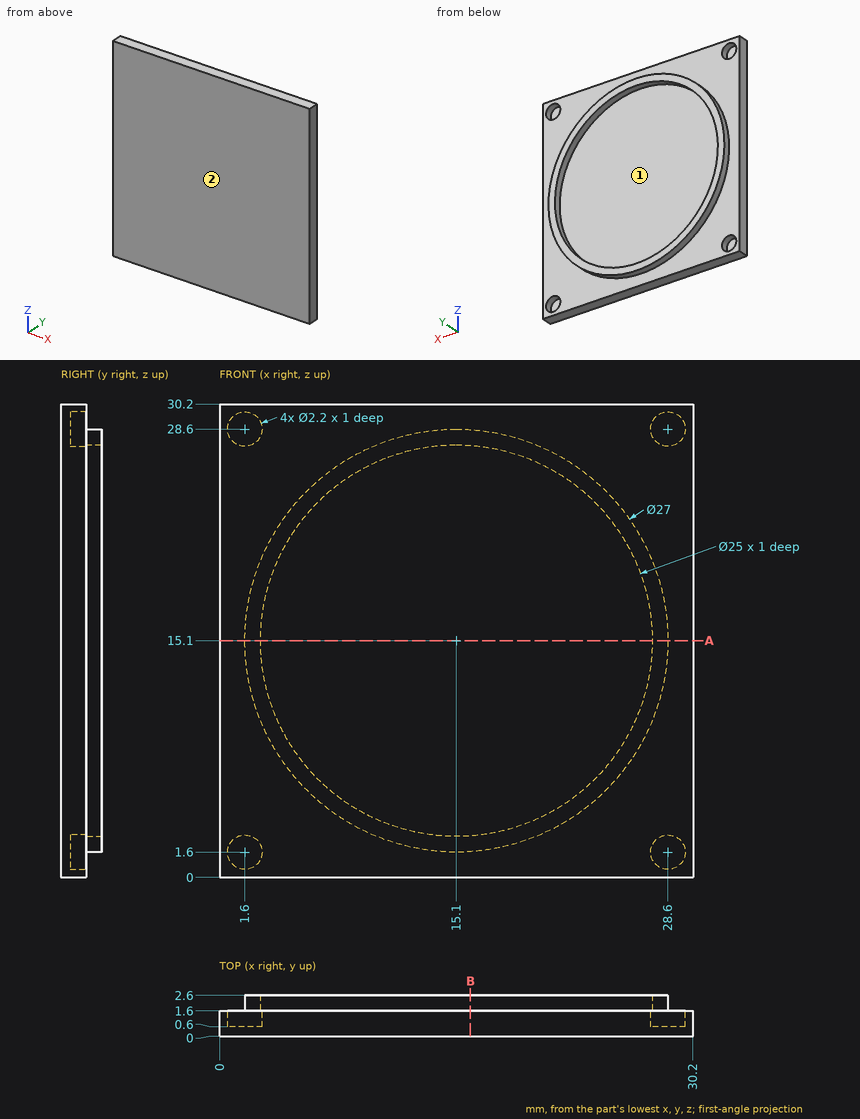
Geometry: see drawing. Coordinates: mm, zero at the bounding-box minimum. Coordinates: 2 decimals unless noted, no trailing zeros. Order: outer loops, then holes, each group sorted by start corner. A loop starts at its lowest first (then second) coordinate and runs counter-clockwise, first axis right, second up. Notation, with made-up numbers: (-16, 32) -> (7, 32) arc R14 ccw to (7, 37) -> close; hole circle Ø3 at (58, 33). An arc over 180 degrees is marked (long way). Write each question's results on one line, items separated by ' | '. Start each with the question number.
1) Cut plane B-B, the plane x = 16. Output: boundary loops of the cut face in (y, z), and give its area (3 significant figures).
2) Mould query, pull axis X, two halves, no side actions, for the marked faces 1 and 2. Classes: released by +X, released by -X, zero draft, split by the parting line, or undercut.
3) Cut plane A-A, the plane z = 15.1. Output: boundary loops of the cut face in (x, y).
4) Material intervals for line 1 along X through (y, z) = (1.1, 1.6); line 2 along Y through (x, z) = (11, 12); line 3 along Z through (x, y) = (2, 1), sorted ascending.
5) First-contact query: pin 1 (7.5 mm diameter, centred on x = 20, z = 18, fed in from +Y); pin 2 (1.3 mm diameter, centred on x = 1.6, z = 1.6, fed in from +Y). Flat tips, straight axial feed; report the tip coordinate or a pass-through.
Checks:
1) outline: (0, 0) -> (1.6, 0) -> (1.6, 1.63) -> (2.6, 1.63) -> (2.6, 2.63) -> (1.6, 2.63) -> (1.6, 27.57) -> (2.6, 27.57) -> (2.6, 28.57) -> (1.6, 28.57) -> (1.6, 30.2) -> (0, 30.2) -> close | area: 50.3 mm^2
2) face 1: undercut | face 2: zero draft
3) outline: (0, 0) -> (30.2, 0) -> (30.2, 1.6) -> (28.6, 1.6) -> (28.6, 2.6) -> (27.6, 2.6) -> (27.6, 1.6) -> (2.6, 1.6) -> (2.6, 2.6) -> (1.6, 2.6) -> (1.6, 1.6) -> (0, 1.6) -> close
4) line 1: 0 to 0.5, 2.7 to 27.5, 29.7 to 30.2 | line 2: 0 to 1.6 | line 3: 0 to 0.58, 2.62 to 27.58, 29.62 to 30.2
5) pin 1: y = 1.6 | pin 2: y = 0.6
